Build history of the part. All positions in model axes, mm. A direction names the side the tool comes from. Round coordinates to 2 decimals unless told otherwise and drop trailing zeros. Write each loop counter-clockwise with the first axis right and the second up, starting at its lowest first coordinate (ties: lowest second). Pieces come first, ordered by that corner, then holes. Notation, with made-up numbers: M 38,31 L 49,31 A20 cw 49,66 Z; hole C 76.25,14.25 d11. An arc over 180 degrees is marked long. Use a Markdown table: item, result.
Autodesk Inventor part; units mm, degrees
ref_plane "YZ Plane" through (0, 0, 0) normal (1, 0, 0) x (0, 1, 0)
ref_plane "XZ Plane" through (0, 0, 0) normal (0, 1, 0) x (-1, 0, 0)
ref_plane "XY Plane" through (0, 0, 0) normal (0, 0, 1) x (1, 0, 0)
sketch "スケッチ1" plane through (0, 0, 0) normal (0, 0, 1) x (1, 0, 0)
  line L0 (0, 0) -> (16, 0)
  line L1 (16, 0) -> (16, 1.5)
  line L2 (16, 1.5) -> (0, 1.5)
  line L3 (0, 1.5) -> (0, 0)
  line L4 (0, 0) -> (0, 2.75)
  line L5 (0, 0) -> (-2, 0)
  line L6 (-2, 0) -> (0, 0)
  line L7 (-2, 0) -> (-2, 1.15)
  arc A0 (0, 2.75) -> (-2, 1.15) centre (-0.0403, 0.7504) ccw
  dimension "d0" = 1.5
  dimension "d1" = 16
  dimension "d3" = 2
  dimension "d4" = 2.75
  dimension "d5" = 1.15
  dimension "d6" = 2
revolve "回転1" add sketch "スケッチ1" angle 360 about axis through (-2, 0, 0) along (1, 0, 0)
thread "ねじ1"
sketch "スケッチ2" plane through (-2, 0, 0) normal (-1, 0, 0) x (0, 0, 1)
  circle A0 centre (0, 0) radius 1.15
  line L0 (-0.575, 0.9959) -> (0.575, 0.9959)
  line L1 (0.575, 0.9959) -> (1.15, 0)
  line L2 (1.15, 0) -> (0.575, -0.9959)
  line L3 (0.575, -0.9959) -> (-0.575, -0.9959)
  line L4 (-0.575, -0.9959) -> (-1.15, 0)
  line L5 (-1.15, 0) -> (-0.575, 0.9959)
  dimension "d10" = 1.15
  dimension "d11" = 1.9919
extrude "押し出し1" cut sketch "スケッチ2" against normal blind 1.4 contours L2 L3 L4 L5 L0 L1
fillet "フィレット1" radius 0.2 6 edges at (-0.6, 0.9959, 0) (-0.6, 0.498, 0.8625) (-0.6, 0.498, -0.8625) (-0.6, -0.498, -0.8625) (-0.6, -0.9959, 0) (-0.6, -0.498, 0.8625)
fillet "フィレット2" radius 0.1 1 edges at (0, -1.5, 0)
fillet "フィレット3" radius 0.1 1 edges at (16, -1.5, 0)
properties part number "ネジボタンM3L16" material "鋼"
Q1. Drill centre lines: L1, parallel to Z at x = 0.75, y = -1.25; L2, parallel to X at y = -0.05, z = -0.3; L3, parallel to X at y = -1.5, z = 1.85. Where is each one in solid material? Low to high.
Response values:
| item | result |
|---|---|
| L1 | z = -0.83 to 0.83 |
| L2 | x = -0.6 to 16 |
| L3 | x = -1.2 to 0 |
Q2. Two-plate mould, pull along Y, no slides. Class faces 3 (the flat face through (0, 2, 0)), 4 (the cylindrical face through (7.89, -1.5, -0.07)), 5 (the flat face through (-1, -0.996, 0)): +Y half, -Y half, draft (parallel to the pull), parting line (faces both ways), or undercut.
Response values:
| item | result |
|---|---|
| face 3 | draft |
| face 4 | parting line |
| face 5 | undercut |
Q3. Drop flat-ended pins along their axis: P1, Ø2, axis at y = -2, z = -2, coming from the -X side; P2, Ø0.5, axis at y = 0, z = 0, coming from the -X side; P3, Ø1.3, axis at x = -1.5, z = 0, coming from the +Y side. Give the stop position or say it passes through.
Response values:
| item | result |
|---|---|
| P1 | stops at x = -1.72 |
| P2 | stops at x = -0.6 |
| P3 | stops at y = 2.58 |
Q4. Which spindle directions (+Z, -Z, +X, -X, +Y, -Y) get a long thin tool onto all of the face, cutting with end or side? Do faces 1 (the flat face through (-1, 0.996, 0)), 2 (the flat face through (16, 0, 0)). Say none if no direction does.
Response values:
| item | result |
|---|---|
| face 1 | -X |
| face 2 | +Z, -Z, +X, +Y, -Y |
Q5. Cut at A-A on x = 14. Give the cut face in (y, z).
Response values:
| item | result |
|---|---|
| outline | C 0,0 d3 |
